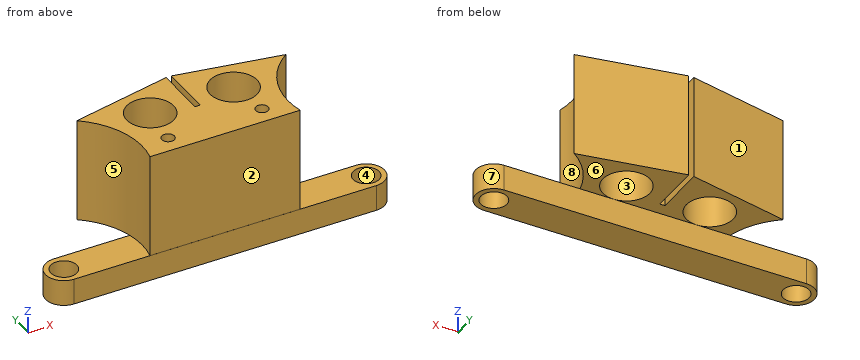
from build123d import *

# Parameters (mm, degrees)
SKETCH_R        = 2.5
PAD_DEPTH       = 5
PAD001_DEPTH    = 20
SKETCH002_R     = 1.2
POCKET_DEPTH    = 10
SKETCH003_R     = 4.5
POCKET001_DEPTH = 25.001


with BuildPart() as part:
    # Sketch → Pad (new body)
    with BuildSketch(Plane.XY):
        with BuildLine():
            ThreePointArc((0, 3.5), (-3.5, 0), (0, -3.5))
            Line((57.98, -3.5), (0, -3.5))
            ThreePointArc((57.98, -3.5), (61.48, 0), (57.98, 3.5))
            Line((0, 3.5), (57.98, 3.5))
        make_face()
        Circle(SKETCH_R, mode=Mode.SUBTRACT)
        with Locations((57.98, 0)):
            Circle(SKETCH_R, mode=Mode.SUBTRACT)
    extrude(amount=PAD_DEPTH)

    # Sketch001 (on Face8 of Pad) → Pad001 (join)
    with BuildSketch(Plane.XY.offset(5)):
        with BuildLine():
            Line((29.489935, 16), (29.489935, 6))
            Line((28.489935, 6), (29.489935, 6))
            Line((28.489935, 6), (28.489935, 15.99995))
            Line((9.108103, 11.918157), (28.489935, 15.99995))
            ThreePointArc((14.587373, -3.494502), (14.133535, 5.024439), (9.108103, 11.918157))
            Line((14.587373, -3.494502), (43.392665, -3.494502))
            ThreePointArc((49.388809, 12.296038), (43.956926, 5.32496), (43.392665, -3.494502))
            Line((29.489935, 16), (49.388809, 12.296038))
        make_face()
    extrude(amount=PAD001_DEPTH)

    # Sketch002 (on Face18 of Pad001) → Pocket (cut)
    with BuildSketch(Plane.XY.offset(25)):
        with Locations((20, 0)):
            Circle(SKETCH002_R)
        with Locations((38, 0)):
            Circle(SKETCH002_R)
    extrude(amount=-POCKET_DEPTH, mode=Mode.SUBTRACT)

    # Sketch003 (on Face18 of Pocket) → Pocket001 (cut, through all)
    with BuildSketch(Plane.XY.offset(25)):
        with Locations((21, 8)):
            Circle(SKETCH003_R)
        with Locations((37, 8)):
            Circle(SKETCH003_R)
    extrude(amount=-POCKET001_DEPTH, mode=Mode.SUBTRACT)


solid = part.part
Geometry: final body of the model. Coordinates: model frame, mm. Face numbers are marked on the shaded views. A direction names the side the tool comes from. Coordinates: 2 decimals unless noted, no trailing zeros. Loops run counter-clockwise (first coordinate to the right, second up) from the corner with the lowest first, then second, coordinate; pieces in that order, holes last. Notation, with made-up numbers: (35.25, 14) - (71.25, 14) arc R24 ccw to (71.25, 24) - close; hole circle Ø11 at (-2, -29.5). An arc over 180 degrees is marked (long way). One line per question, with ' | ' between items. Start each with the question number.
(1) Reachability of the marked faces 5, 6, 7 and 8 from +Z, -Z, +X, -X, +Y, -Y: full face, straight path, thin tool, end or side. Return the list, or none.
(2) Ray query, L1, parallel to X at y = 10.75, z = 12.5; L2, parallel to Y at x = 21, z = 19; L3, parallel to Y at x = 37, z = 17. Return the intervals inside material, ascending. Write a range as from..to.
(3) Cut plane D-D on y = 9. Output: boundary loops of the cut face in (x, z), and give its area (3 significant figures).
(4) Cut plane B-B on z = 21.5. Output: boundary loops of the cut face in (x, y), and give its area (3 significant figures).
(5) First-contact query: pin 1 (12 mm diameter, centred on x = 36, z = 17.5, fed in from +Y); pin 2 (4 mm diameter, centred on x = 27.5, y = 9.5, fed in from -Z); pin 3 (4 mm diameter, centred on x = 29.5, z = 2.5, fed in from +Y). Flat tips, straight axial feed; report the tip coordinate or a pass-through.
(6) Cut plane C-C on x = 48.5. Output: boundary loops of the cut face in (y, z), and give its area (3 significant figures).
(7) Draft query along X for the marked faces 1, 2, 3 and 4. Return one class per face: +X half, -X half, draft (parallel to the pull), parting line (faces both ways), or undercut.
(8) Cut plane A-A on z = 12. Output: boundary loops of the cut face in (x, y), and give its area (3 significant figures).
Here are the results:
1) face 5: +Z, -X | face 6: -Z, +X, -X, +Y | face 7: +Z, -Z, +X | face 8: +Z, +X
2) L1: 10.46..17.44, 24.56..28.49, 29.49..33.44, 40.56..47.52 | L2: -3.49..-0.66, 0.66..3.5, 12.5..14.42 | L3: -3.49..-0.66, 0.66..3.5, 12.5..14.6
3) outline: (12, 5) - (16.61, 5) - (16.61, 25) - (12, 25) - close; (25.39, 5) - (28.49, 5) - (28.49, 25) - (25.39, 25) - close; (29.49, 5) - (32.61, 5) - (32.61, 25) - (29.49, 25) - close; (41.39, 5) - (45.98, 5) - (45.98, 25) - (41.39, 25) - close | area: 309 mm²
4) outline: (9.11, 11.92) arc R15 cw to (14.59, -3.49) - (43.39, -3.49) arc R15 cw to (49.39, 12.3) - (29.49, 16) - (29.49, 6) - (28.49, 6) - (28.49, 16) - close; hole circle Ø9 at (21, 8); hole circle Ø2.4 at (20, 0); hole circle Ø9 at (37, 8); hole circle Ø2.4 at (38, 0) | area: 416 mm²
5) pin 1: y = 15.91 | pin 2: z = 5 | pin 3: y = 3.5
6) outline: (-3.5, 0) - (3.5, 0) - (3.5, 5) - (-3.5, 5) - close; (11.62, 5) - (12.46, 5) - (12.46, 25) - (11.62, 25) - close | area: 51.7 mm²
7) face 1: -X half | face 2: draft | face 3: undercut | face 4: undercut
8) outline: (9.11, 11.92) arc R15 cw to (14.59, -3.49) - (43.39, -3.49) arc R15 cw to (49.39, 12.3) - (29.49, 16) - (29.49, 6) - (28.49, 6) - (28.49, 16) - close; hole circle Ø9 at (21, 8); hole circle Ø9 at (37, 8) | area: 425 mm²
